Autodesk Inventor part; units mm, degrees
ref_plane "YZ Plane" through (0, 0, 0) normal (1, 0, 0) x (0, 1, 0)
ref_plane "XZ Plane" through (0, 0, 0) normal (0, 1, 0) x (-1, 0, 0)
ref_plane "XY Plane" through (0, 0, 0) normal (0, 0, 1) x (1, 0, 0)
sketch "Sketch1" plane through (0, 0, 0) normal (0, 0, 1) x (1, 0, 0)
  line L0 (0, 0) -> (0, 60)
  line L1 (0, 60) -> (9, 60) construction
  line L2 (9, 60) -> (25, 0) construction
  line L3 (25, 0) -> (0, 0) construction
  line L4 (28.2341, -0.4847) -> (11.3048, 63)
  line L5 (11.3048, 63) -> (-3, 63)
  line L6 (-3, 63) -> (-3, -3)
  line L7 (-3, -3) -> (26.3016, -3)
  line L8 (0, 60) -> (0, 63)
  line L9 (0, 0) -> (0, -3)
  arc A0 (26.3016, -3) -> (28.2341, -0.4847) centre (26.3016, -1) ccw
  point P0 (28.9048, -3)
  dimension "d0" = 9
  dimension "d1" = 25
  dimension "d2" = 60
  dimension "d5" = 3
  dimension "d19" = 2
extrude "Extrusion1" add sketch "Sketch1" along normal blind 2 contours L0 L8 L5 L4 A0 L7 L9
chamfer "Chamfer1" distance 1.5 angle 45 4 edges at (19.7695, 31.2577, 2) (27.8876, -2.2185, 2) (13.1508, -3, 2) (5.6524, 63, 2)
sketch "Sketch2" plane through (0, 0, 2) normal (0, 0, 1) x (1, 0, 0)
  line L0 (6, -14.251) -> (6, 80.2953) construction
  line L1 (0, 61.5) -> (0, -1.5)
  circle A0 centre (6, 7) radius 2.1
  circle A1 centre (6, 42) radius 2.1
  line L2 (0, -3) -> (26.3016, -3)
  point P0 (0, 0)
  point P1 (28.8571, -3)
  dimension "d9" = 6
  dimension "d10" = 4.2
  dimension "d11" = 4.2
  dimension "d12" = 10
  dimension "d13" = 45
extrude "Extrusion2" cut sketch "Sketch2" against normal up to surface (2 mm away)
chamfer "Chamfer2" distance 2 angle 45 2 edges at (3.9, 42, 2) (3.9, 7, 2)
equation "\"d11\" = d10"
properties part number "spazzola - appoggio"
Could you check a few things on this model? Use its own coordinates, in mm. Give positions to 0.01 mm unless a question says otherwise; leave off trailing zeros. Order: outer loops, then holes, each group sorted by start corner. A loop starts at its lowest first (then second) coordinate and runs counter-clockwise, first axis right, second up. Notation, with made-up numbers: (-22, -22.5) - (3, -22.5) arc R25 ccw to (3, -2.5) - close; hole circle Ø4 at (77.25, 21). An arc over 180 degrees is marked (long way). One line per question, with ' | ' between items. Start each with the question number.
Item 1: I need wall thicknesses on probe 1 along Y at (x, z) = (6, 0.05); probe 2 along Y at (x, z) = (8.5, 1.45); probe 3 along X at (y, z) = (44, 1.8). Which ranges of each line are inside material? Lowest first, please. Write a range as [from, to].
Item 2: I want a section at C-C on z = 1.2. Write out the boundary of the cut face in (x, y).
Item 3: I'm going to push flat-ended pins straight in: pin 1 Ø5 at (x, y) = (6, 7) entering from +Z; pin 2 Ø5.5 at (x, y) = (6, 42) entering from +Z. Where does each tip first touch, or does it pass through?
Item 4: I want a section at A-A on x = 6. Give the number of separate pieces and of enclosed holes in the cut face, then the cut area to 3 significant figures.
Verdict:
1) probe 1: [-3, 4.85], [9.15, 39.85], [44.15, 63] | probe 2: [-2.05, 4.48], [9.52, 39.48], [44.52, 62.05] | probe 3: [0, 2.65], [9.35, 15.03]
2) outline: (0, -2.3) - (26.3, -2.3) arc R1.3 ccw to (27.56, -0.67) - (10.77, 62.3) - (0, 62.3) - close; hole circle Ø6.6 at (6, 7); hole circle Ø6.6 at (6, 42)
3) pin 1: z = 0.4 | pin 2: z = 0.65
4) separate pieces: 3 | enclosed holes: 0 | area: 105 mm^2
